Can you work these out from the drawing? Everything is in mm from the part's minimum corner. A direction names the side the tool comes from. Give positions to 0.01 mm unless a question says otherwise; leave off trailing zeros. Loops run counter-clockwise (first coordinate to the right, second up) from the corner with the lowest first, then second, coordinate; pieces in that order, holes last.
Q1. If we section it at A-A (x = 4.7): Please give me the cut outline in (y, z).
Q2. If we section it at B-B (z = 12): Please give me the cut outline in (x, y).
Q3. For the marked faces 1, 2 and 3, which set-ups out of +Z, -Z, +X, -X, +Y, -Y let a thin tool reach every point of the face, with its end or its side?
Q4. If we section it at C-C (y = 18): Please give me the cut outline in (x, z), plus the area to 3 significant figures.
Q5. I need wall thicknesses on line 1 (Y direction, x = 1.25, z = 5.5); line 2 (Y direction, x = 2.5, z = 8.5); line 3 (X direction, y = 23, z = 11.25). Which ranges of each line are inside material? Lowest first, please.
Q6. Will these pins go through, and if not, where does the flat tip stop? P1, Ø1.6, axis at y = 23.5, z = 12.5, coming from the -X side; P2, Ø5, axis at y = 10, z = 5, coming from the +X side; P3, Ø1, axis at x = 5, z = 1, coming from the +Y side.
Q7. We'd pull the mould along Z, two halves only. Please class the marked faces 4, 5 and 6: +Z half, -Z half, draft (parallel to the pull), parting line (faces both ways), or undercut.
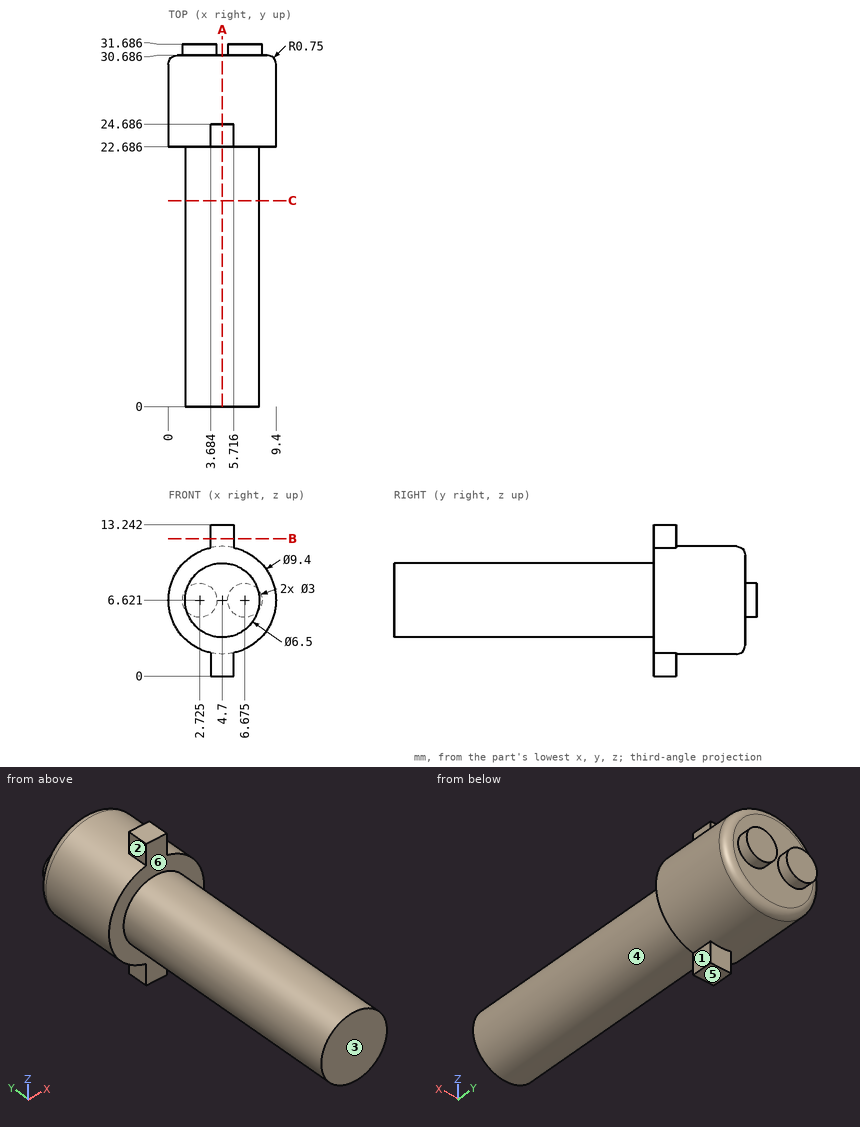
Check sheet entries:
1. outline: (0, 3.37) - (22.69, 3.37) - (22.69, 0) - (24.69, 0) - (24.69, 1.92) - (29.94, 1.92) arc R0.75 ccw to (30.69, 2.67) - (30.69, 10.57) arc R0.75 ccw to (29.94, 11.32) - (24.69, 11.32) - (24.69, 13.24) - (22.69, 13.24) - (22.69, 9.87) - (0, 9.87) - close
2. outline: (3.68, 22.69) - (5.72, 22.69) - (5.72, 24.69) - (3.68, 24.69) - close
3. face 1: -Z, +X, +Y, -Y
3. face 2: +Z, -X, +Y, -Y
3. face 3: +Z, -Z, +X, -X, -Y
4. outline: circle Ø6.5 at (4.7, 6.62)
4. area: 33.2 mm2
5. line 1: y = 22.69 to 30.69
5. line 2: y = 0 to 30.69
5. line 3: x = 3.68 to 5.72
6. P1: stops at x = 3.68
6. P2: stops at x = 7.95
6. P3: stops at y = 24.69
7. face 4: parting line
7. face 5: -Z half
7. face 6: draft
